Model file for the job. Use its own axes, mm. A direction names the side the tool comes from. Coordinates: 2 decimals unless noted, no trailing zeros. Order: outer loops, then holes, each group sorted by start corner. A loop starts at its lowest first (then second) coordinate and runs counter-clockwise, first axis right, second up. Notation, with made-up numbers: (66, 39) - (123, 39) arc R11 ccw to (123, 54) - close; hole circle Ø5 at (59.5, 38.5). An arc over 180 degrees is marked (long way). Put each result on its own line as item: value. Start each with the question number.
```python
from build123d import *

# Parameters (mm, degrees)
SKICA2_R                 = 19
SKICA2_R_2               = 7
P_IDAT_VYSUNUT_M1_DEPTH  = 14
ZAOBLIT1_R               = 3
SKICA3_R                 = 33
SKICA3_R_2               = 19
ODEBRAT_VYSUNUT_M1_DEPTH = 2
ZKOSEN_1_SIZE            = 2
ZAOBLIT2_R               = 2
KRUHOV_POLE1_COUNT       = 4


with BuildPart() as part:
    # Skica1 → Rotovat1 (revolve)
    with BuildSketch(Plane.XY, mode=Mode.PRIVATE) as rotovat1_sk:
        Polygon((0, 19), (0, 32.5), (-4, 32.5), (-4, 30), (-28, 25), (-28, 22.5), (-24, 22.5), (-24, 19), align=None)
    revolve(rotovat1_sk.sketch.rotate(Axis((-37.430213862, 0, 0), (1, 0, 0)), 90), axis=Axis((-37.430213862, 0, 0), (1, 0, 0)))

    # Skica2 → Přidat vysunutím1 (add)
    with BuildSketch(Plane(origin=(0, 0, 0), x_dir=(0, 0, -1), z_dir=(1, 0, 0))):
        with BuildLine():
            Line((-33.336202543, -18.24), (-12.281758832, -56.72))
            ThreePointArc((-12.281758832, -56.72), (0, -64), (12.281758832, -56.72))
            Line((12.281758832, -56.72), (33.336202543, -18.24))
            ThreePointArc((33.336202543, -18.24), (38, 0), (33.336202543, 18.24))
            Line((33.336202543, 18.24), (12.281758832, 56.72))
            ThreePointArc((12.281758832, 56.72), (0, 64), (-12.281758832, 56.72))
            Line((-12.281758832, 56.72), (-33.336202543, 18.24))
            ThreePointArc((-33.336202543, 18.24), (-38, 0), (-33.336202543, -18.24))
        make_face()
        with Locations(Location((0, 0, 0), (0, 0, 180))):
            Circle(SKICA2_R, mode=Mode.SUBTRACT)
        with Locations((0, 50)):
            Circle(SKICA2_R_2, mode=Mode.SUBTRACT)
        with Locations((0, -50)):
            Circle(SKICA2_R_2, mode=Mode.SUBTRACT)
    extrude(amount=P_IDAT_VYSUNUT_M1_DEPTH)

    # Zaoblit1
    zaoblit1_edges = [part.edges().sort_by_distance(p)[0] for p in [
        (-4, 0, -30),
    ]]
    fillet(zaoblit1_edges, radius=ZAOBLIT1_R)

    # Skica3 → Odebrat vysunutím1 (cut)
    with BuildSketch(Plane(origin=(14, 0, 0), x_dir=(0, 0, -1), z_dir=(1, 0, 0))):
        Circle(SKICA3_R)
        with Locations(Location((0, 0, 0), (0, 0, 180))):
            Circle(SKICA3_R_2, mode=Mode.SUBTRACT)
    extrude(amount=-ODEBRAT_VYSUNUT_M1_DEPTH, mode=Mode.SUBTRACT)

    # Zkosení1
    zkosen_1_edges = [part.edges().sort_by_distance(p)[0] for p in [
        (-24, 0, -19),
    ]]
    chamfer(zkosen_1_edges, length=ZKOSEN_1_SIZE)

    # Zaoblit2
    zaoblit2_edges = [part.edges().sort_by_distance(p)[0] for p in [
        (0, 0, -32.5),
        (-28, 0, -25),
    ]]
    fillet(zaoblit2_edges, radius=ZAOBLIT2_R)

    # Skica6 → M5 závit1 (revolve, cut)
    with BuildSketch(Plane(origin=(12, 0, 26), x_dir=(0, 0, -1), z_dir=(0, 1, 0))):
        Polygon((0, 0), (0, 11.2618073), (2.1, 10), (2.1, 0), align=None)
    m5_z_vit1 = revolve(axis=Axis((18.35, 0, 26), (-1, 0, 0)), mode=Mode.SUBTRACT)

    # Kruhové pole1: M5 závit1 ×4 about axis
    kruhov_pole1_axis = Axis((0, 0, 0), (1, 0, 0))
    for i in range(1, KRUHOV_POLE1_COUNT):
        add(m5_z_vit1.rotate(kruhov_pole1_axis, i * 360 / KRUHOV_POLE1_COUNT), mode=Mode.SUBTRACT)


solid = part.part
```
Item 1: Wall check: line 1 along Z through (x, y) = (-1, -6.5); line 2 along Y through (x, z) = (-5, 0); line 3 along Y through (x, z) = (4.5, 11). Give the ranges that are in metal, low to high.
Item 2: Slice it at D-D, the plane z = -5. Give the number of separate pieces and of enclosed holes in the cut face, plus the area to 3 significant figures.
Item 3: Slice it at A-A, the plane y = -54. Give the cut face in (x, z), plus the area to 3 significant figures.
Item 4: Flat gauge pins, fed straight in: pin 1 Ø8.5 at (y, z) = (-50, 0) entering from +X; pin 2 Ø2.5 at (y, z) = (26, 0) entering from -X; pin 3 Ø12 at (x, y) = (-7, -15.5) entering from +Z; pin 4 Ø4 at (y, z) = (34.5, -26) entering from -X. Where does each tip first touch, or does it go through?
Item 5: Slice it at C-C, the plane x = -14. Give the cut face in (y, z).
Item 6: 3-axis set-ups, long thin cutter, end or side, ignore diameter. For faces 1 (the face through (7, 0, -38)), 2 (the face through (7.07, 1.863, 25.031)): which of +Z, -Z, +X, -X, +Y, -Y reach the whole face in a straight line?
Item 7: Pull direction Z, two halves, no side cores. Call faces 3 (the face through (-3.01, -9.76, 31)), 4 (the face through (7, 0, 38)), 5 (the face through (-24, 20, -7)): pulls with the +Z half, pulls with the -Z half, needs draft (parallel to the pull), parting line crosses it, or undercut.
Item 8: Slice it at B-B, the plane x = 7. Give the cut face in (y, z).
Here are the results:
1. line 1: z = -32.12 to -17.85, 17.85 to 32.12
1. line 2: y = -30.2 to -19, 19 to 30.2
1. line 3: y = -58.66 to -15.49, 15.49 to 58.66
2. separate pieces: 4
2. enclosed holes: 0
2. area: 1,420 mm^2
3. outline: (0, -13.77) - (14, -13.77) - (14, -5.74) - (0, -5.74) - close; (0, 5.74) - (14, 5.74) - (14, 13.77) - (0, 13.77) - close
3. area: 225 mm^2
4. pin 1: passes through
4. pin 2: stops at x = -27.45
4. pin 3: stops at z = 30.82
4. pin 4: stops at x = 0
5. outline: circle Ø55.83 at (0, 0); hole circle Ø38 at (0, 0)
6. face 1: -Z, +X, -X
6. face 2: +X
7. face 3: parting line crosses it
7. face 4: pulls with the +Z half
7. face 5: undercut
8. outline: (-56.72, -12.28) - (-18.24, -33.34) arc R38 ccw to (18.24, -33.34) - (56.72, -12.28) arc R14 ccw to (56.72, 12.28) - (18.24, 33.34) arc R38 ccw to (-18.24, 33.34) - (-56.72, 12.28) arc R14 ccw to start; hole circle Ø14 at (-50, 0); hole circle Ø4.2 at (-26, 0); hole circle Ø38 at (0, 0); hole circle Ø4.2 at (0, -26); hole circle Ø4.2 at (0, 26); hole circle Ø4.2 at (26, 0); hole circle Ø14 at (50, 0)
